CAD build for the part. Positions are in the model's coordinates, mm. A direction names the side the tool comes from. Give positions to 0.01 mm unless a question says otherwise; leave off trailing zeros. Write each loop counter-clockwise with the first axis right and the second up, starting at its lowest first coordinate (ties: lowest second). Pieces come first, ordered by that corner, then holes. Notation, with made-up numbers: (31.25, -16.75) - (59.25, -16.75) arc R30 ccw to (59.25, 13.25) - close; hole circle Ø2 at (66, 23). An arc over 180 degrees is marked (long way). Answer as a JSON object with one key per item and string values.
from build123d import *

# Parameters (mm, degrees)
F1_DEPTH = 25


with BuildPart() as f1:
    # F0 (on Front) → F1 (new body)
    with BuildSketch(Plane.XZ):
        Polygon((-150, 0), (0, 0), (150, 0), (206.01979, -597.379095), (226.01979, -597.379095), (166.723986, 34.934477), (146.723986, 34.934477), (148.124481, 20), (15, 20), (15, 10), (0, 10), (-15, 10), (-15, 20), (-15.339315, 20), (-148.124481, 20), (-146.723986, 34.934477), (-166.723986, 34.934477), (-226.01979, -597.379095), (-206.01979, -597.379095), align=None)
    extrude(amount=F1_DEPTH)


solid = f1.part
(1) Probe L1, parallel to Z at x = 89, y = -9; L2, parallel to X at y = -5.75, z = -243; L3, parallel to X at y = -6.5, z = -175. List the from-to ranges inside material, lowest first. Write a range as [from, to].
Answer key:
{"L1": "z = [0, 20]", "L2": "x = [-192.79, -172.79], [172.79, 192.79]", "L3": "x = [-186.41, -166.41], [166.41, 186.41]"}
(2) Saw through at B-B, the plane z = -463. Give the cut face in (x, y), and give its area (4 significant figures).
Answer key:
{"outline": "(-213.42, -25) - (-193.42, -25) - (-193.42, 0) - (-213.42, 0) - close; (193.42, -25) - (213.42, -25) - (213.42, 0) - (193.42, 0) - close", "area": "1,000 mm²"}
(3) Saw through at D-D, the plane x = 184. Give the cut face in (y, z), and give its area (3 significant figures).
Answer key:
{"outline": "(-25, -362.57) - (0, -362.57) - (0, -149.29) - (-25, -149.29) - close", "area": "5,330 mm²"}
(4) 3-axis set-ups, long thin cutter, end or side, ignore diameter. For faces 1 (the face through (0, -12, 10)), 2 (the face through (-178.4, -12.32, -302.87)), 3 (the face through (-147.434, -12.325, 27.363)): which of +Z, -Z, +X, -X, +Y, -Y reach the whole face in a straight line?
Answer key:
{"face 1": "+Z, +Y, -Y", "face 2": "-Z, +Y, -Y", "face 3": "+Y, -Y"}
(5) Pull direction X, two halves, no side cores. Call faces 4 (the face through (82, -12, 20)), 5 (the face through (-195.957, -12.325, -276.796)), 6 (the face through (196.787, -12.325, -285.649)), 7 (the face through (157, -12, 34.934)): pulls with the +X half, pulls with the -X half, needs draft (parallel to the pull), parting line crosses it, or undercut.
Answer key:
{"face 4": "undercut", "face 5": "pulls with the -X half", "face 6": "pulls with the +X half", "face 7": "needs draft"}
(6) Saw through at A-A, the plane y = -17. Give the cut face in (x, z).
Answer key:
{"outline": "(-226.02, -597.38) - (-206.02, -597.38) - (-150, 0) - (150, 0) - (206.02, -597.38) - (226.02, -597.38) - (166.72, 34.93) - (146.72, 34.93) - (148.12, 20) - (15, 20) - (15, 10) - (-15, 10) - (-15, 20) - (-148.12, 20) - (-146.72, 34.93) - (-166.72, 34.93) - close"}
(7) Saw through at C-C, the plane x = -97. Give the cut face in (y, z).
Answer key:
{"outline": "(-25, 0) - (0, 0) - (0, 20) - (-25, 20) - close"}
(8) Flat gauge pins, fed straight in: P1, Ø5, axis at y = -17, z = -53, coming from the -X side; P2, Ø5, axis at y = -11.5, z = 15, coming from the +X side; P3, Ø7.5, axis at x = 45.5, y = -15, coming from the -Z side. Where does each tip first touch, or does it go through?
Answer key:
{"P1": "stops at x = -175.2", "P2": "stops at x = 168.83", "P3": "stops at z = 0"}
